Geometry: final body of the model. Coordinates: model frame, mm. Face numbers are marked on the shaded views. Give positions to 0.01 mm unless a question says otherwise; leave off trailing zeros. Loops run counter-clockwise (first coordinate to the right, second up) from the corner with the lowest first, then second, coordinate; pieces in that order, holes last.
from build123d import *

# Parameters (mm, degrees)
SKETCH2_R           = 25
SKETCH2_R_2         = 5.1
BOSS_EXTRUDE1_DEPTH = 2.5
SKETCH3_R           = 7.1
SKETCH3_R_2         = 5.1
BOSS_EXTRUDE2_DEPTH = 3
FILLET1_R           = 1
FILLET2_R           = 1


with BuildPart() as part:
    # Sketch2 → Boss-Extrude1 (new body)
    # profile 1 of 2: a face of its own
    with BuildSketch(Plane(origin=(0, 0, 0), x_dir=(1, 0, 0), z_dir=(0, 1, 0))):
        with Locations(Location((0, 0, 0), (0, 0, 270))):
            Circle(SKETCH2_R)
        Circle(SKETCH2_R_2, mode=Mode.SUBTRACT)
    # profile 2 of 2: a face of its own
    with BuildSketch(Plane(origin=(0, 0, 0), x_dir=(1, 0, 0), z_dir=(0, 1, 0))):
        Circle(SKETCH2_R_2)
    extrude(amount=BOSS_EXTRUDE1_DEPTH)

    # Sketch3 → Boss-Extrude2 (add)
    with BuildSketch(Plane(origin=(0, 2.5, 0), x_dir=(1, 0, 0), z_dir=(0, 1, 0))):
        with Locations(Location((0, 0, 0), (0, 0, 270))):
            Circle(SKETCH3_R)
        with Locations(Location((0, 0, 0), (0, 0, 270))):
            Circle(SKETCH3_R_2, mode=Mode.SUBTRACT)
    extrude(amount=BOSS_EXTRUDE2_DEPTH)

    # Fillet1
    fillet1_edges = [part.edges().sort_by_distance(p)[0] for p in [
        (0, 2.5, -5.1),
    ]]
    fillet(fillet1_edges, radius=FILLET1_R)

    # Fillet2
    fillet2_edges = [part.edges().sort_by_distance(p)[0] for p in [
        (0, 2.5, -7.1),
    ]]
    fillet(fillet2_edges, radius=FILLET2_R)


solid = part.part
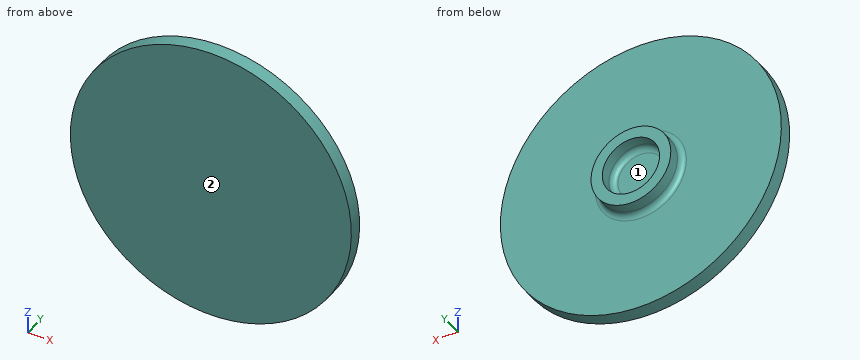
Item 1: Section query C-C on x = -15.5. Return loops of the section in (y, z), plus the area to 3 significant figures.
Values follow:
outline: (0, -19.62) - (2.5, -19.62) - (2.5, 19.62) - (0, 19.62) - close
area: 98.1 mm2
Item 2: Pin query (flat end, axial travel): pin 1 (1 mm diameter, centred on x = 1, y = 2.5, fed in from -Z) (3 decimals); pin 2 (1 mm diameter, centred on y = 3.5, z = 8.5, fed in from +X); pin 3 (6.5 mm diameter, centred on x = 0.5, z = 1, fed in from +Y); pin 4 (9 mm diameter, centred on x = 0, z = 0, fed in from +Y). Return the tip coordinate at first contact, or that it passes through.
Values follow:
pin 1: stops at z = -24.995
pin 2: passes through
pin 3: stops at y = 2.54
pin 4: stops at y = 2.58
Item 3: Section query A-A on z = 0. Return loops of the section in (x, y).
Values follow:
outline: (-25, 0) - (25, 0) - (25, 2.5) - (8.1, 2.5) arc R1 cw to (7.1, 3.5) - (7.1, 5.5) - (5.1, 5.5) - (5.1, 3.5) arc R1 cw to (4.1, 2.5) - (-4.1, 2.5) arc R1 cw to (-5.1, 3.5) - (-5.1, 5.5) - (-7.1, 5.5) - (-7.1, 3.5) arc R1 cw to (-8.1, 2.5) - (-25, 2.5) - close
Item 4: Section query B-B on x = 0. Return loops of the section in (y, z).
Values follow:
outline: (0, -25) - (2.5, -25) - (2.5, -8.1) arc R1 cw to (3.5, -7.1) - (5.5, -7.1) - (5.5, -5.1) - (3.5, -5.1) arc R1 cw to (2.5, -4.1) - (2.5, 4.1) arc R1 cw to (3.5, 5.1) - (5.5, 5.1) - (5.5, 7.1) - (3.5, 7.1) arc R1 cw to (2.5, 8.1) - (2.5, 25) - (0, 25) - close
Item 5: Ray query, probe 1 along X at (y, z) = (4.05, 0); probe 2 along Y at (x, z) = (1.5, 22); probe 3 along X at (y, z) = (4.5, -4). Return the intervals inside material, ascending.
Values follow:
probe 1: x = -7.1 to -5.1, 5.1 to 7.1
probe 2: y = 0 to 2.5
probe 3: x = -5.87 to -3.16, 3.16 to 5.87
Item 6: Section query D-D on z = -19. Return loops of the section in (x, y).
Values follow:
outline: (-16.25, 0) - (16.25, 0) - (16.25, 2.5) - (-16.25, 2.5) - close
Item 7: Draft query along Z for the marked faces 1 and 2. Return one class per face: +Z half, -Z half, draft (parallel to the pull), parting line (faces both ways), or undercut.
Values follow:
face 1: undercut
face 2: draft
